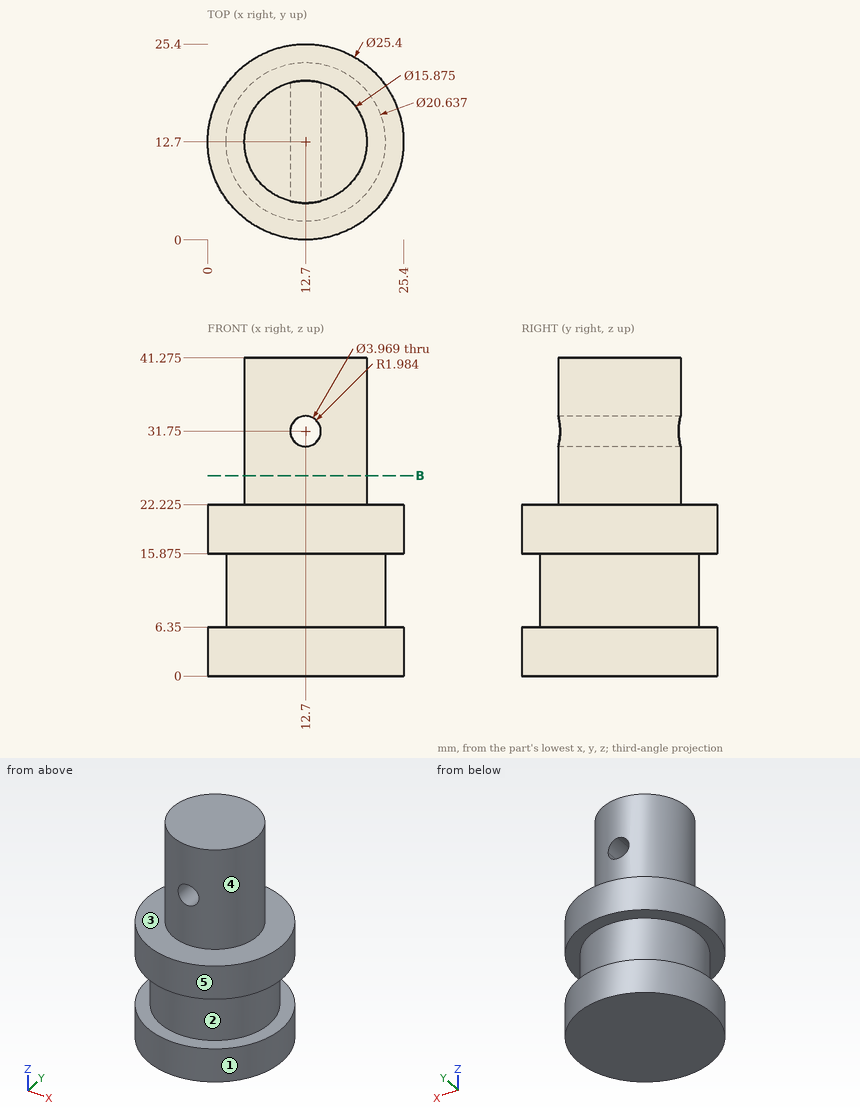
Answer from the drawing. Dimensions are ordinates in mm from the lowest x, y and z of the part. A direction names the side the tool comes from. Give positions to 0.01 mm unless a question says otherwise; leave off trailing zeros. Order: outer loops, then holes, each group sorted by start corner. A loop starts at its lowest first (then second) coordinate and runs counter-clockwise, first axis right, second up. Notation, with made-up numbers: (89, -22.75) - (102, -22.75) arc R24 cw to (102, 13.25) - close; hole circle Ø5 at (-26, 39). An arc over 180 degrees is marked (long way). One line per item, written item: value. Start each with the question number.
1. Each of these flat-tipped pins is pushed along its axis until it touches: pin 1 Ø8 at (x, z) = (9.5, 13.5) entering from -Y; pin 2 Ø6 at (x, z) = (14.5, 36) entering from -Y; pin 3 Ø6 at (y, z) = (12.5, 29) entering from -X; pin 4 Ø2 at (x, z) = (5, 16.5) entering from -Y. Where does it stop, or does it pass through?
2. Consider line 1 (Z direction, x = 12.7, y = 11.75) (1 decimal); line 2 (X direction, y = 11, z = 31.75) (1 decimal); line 3 (X direction, y = 13, z = 31.75) (1 decimal). Determine where each line is inside the solid, lowest interval first.
3. Section B-B, the plane z = 26 is taken. Write down the section's boundary in (x, y) (1 decimal), then the cut area to 3 significant figures.
4. For a pull along Z with two mould halves and no side action, classify the marked faces 1, 2 and 3 as released by +Z, released by -Z, zero draft, split by the parting line, or undercut.
5. Which of the six approach directions +Z, -Z, +X, -X, +Y, -Y give full straight-line access (tool end or side, diameter ignored) to the marked faces 4 and 5?
Filled sheet:
1. pin 1: y = 0
1. pin 2: y = 4.76
1. pin 3: x = 4.76
1. pin 4: y = 1.91
2. line 1: 0 to 29.8, 33.7 to 41.3
2. line 2: 4.9 to 10.7, 14.7 to 20.5
2. line 3: 4.8 to 10.7, 14.7 to 20.6
3. outline: circle Ø15.9 at (12.7, 12.7)
3. area: 198 mm²
4. face 1: zero draft
4. face 2: undercut
4. face 3: released by +Z
5. face 4: +Z
5. face 5: +Z, -Z
